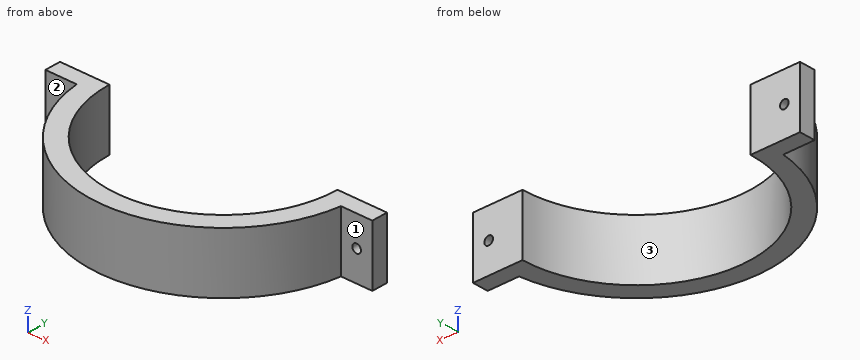
from build123d import *

# Parameters (mm, degrees)
BOSS_EXTRUDE1_DEPTH = 30
SKETCH2_W           = 20
SKETCH2_H           = 8
BOSS_EXTRUDE2_DEPTH = 30
SKETCH3_R           = 2.15265
CUT_EXTRUDE1_DEPTH  = 67.675


with BuildPart() as part:
    # Sketch1 → Boss-Extrude1 (new body)
    with BuildSketch(Plane.XY):
        with BuildLine():
            Line((66.675, 0), (57.15, 0))
            ThreePointArc((57.15, 0), (0, -57.15), (-57.15, 0))
            Line((-57.15, 0), (-66.675, 0))
            ThreePointArc((-66.675, 0), (0, -66.675), (66.675, 0))
        make_face()
    extrude(amount=BOSS_EXTRUDE1_DEPTH)

    # Sketch2 → Boss-Extrude2 (add)
    with BuildSketch(Plane.XY.offset(30)):
        with Locations((71.9125, -4)):
            Rectangle(SKETCH2_W, SKETCH2_H)
        with Locations((-71.9125, -4)):
            Rectangle(SKETCH2_W, SKETCH2_H)
    extrude(amount=-BOSS_EXTRUDE2_DEPTH)

    # Sketch3 → Cut-Extrude1 (cut, through all)
    with BuildSketch(Plane(origin=(0, 0, 0), x_dir=(1, 0, 0), z_dir=(0, 1, 0))):
        with Locations((-74.052910047, -15)):
            Circle(SKETCH3_R)
        with Locations((74.052910047, -15)):
            Circle(SKETCH3_R)
    extrude(amount=-CUT_EXTRUDE1_DEPTH, mode=Mode.SUBTRACT)


solid = part.part
The listing builds one solid part. Answer for the finished solid, in the listing's coordinates (mm). Face numbers are marked on the shaded views. A direction names the side the tool comes from. Round coordinates to 2 decimals unless told otherwise and drop trailing zeros. Write each loop counter-clockwise with the first axis right and the second up, starting at its lowest first coordinate (ties: lowest second). Pieces come first, ordered by that corner, then holes. Notation, with made-up numbers: (-39.5, -24.75) - (-17.5, -24.75) arc R17 cw to (-17.5, -17.75) - close; hole circle Ø4 at (-5, 21). An arc over 180 degrees is marked (long way). Use a Markdown table: item, result. Add a question column.
1. Flat-ended cylindrical pins translate along their axes: P1, Ø10, axis at x = -21.5, z = 25.5, coming from the -Y side; P2, Ø7, axis at x = 74.05, z = 15, coming from the -Y side; P3, Ø1, axis at y = -46.5, z = 21.5, coming from the -X side. Find the tip coordinate at first contact, or state that the pin passes through.
2. The part is cut by section A-A (z = 15). Give the number of separate pieces and of enclosed holes in the cut face, and give its area (3 significant figures).
3. A tool of negligible diameter and unlimited length cuts with its end or side. For the marked faces 1, 2 and 3, from which of +Z, -Z, +X, -X, +Y, -Y can it reach the whole face along a straight path? Write none if from no direction.
4. The part is cut by section B-B (y = -22). Write down the section's boundary in (x, z), and give its area (3 significant figures).
5. Consider line 1 (X direction, y = -2.75, z = 15); line 2 (X direction, y = -3.75, z = 15); line 3 (X direction, y = -29, z = 28.25). Determine where each line is inside the solid, lowest interval first.
6. The part is cut by section D-D (y = -14). Write down the section's boundary in (x, z), and give its area (3 significant figures).
Reported:
| question | item | result |
|---|---|---|
| 1 | P1 | y = -64.6 |
| 1 | P2 | y = -8 |
| 1 | P3 | x = -48.27 |
| 2 | separate pieces | 3 |
| 2 | enclosed holes | 0 |
| 2 | area | 2,030 mm^2 |
| 3 | face 1 | +Z, -Z, +X, -Y |
| 3 | face 2 | +Z, -Z, -X, -Y |
| 3 | face 3 | +Z, -Z, +Y |
| 4 | outline | (-62.94, 0) - (-52.75, 0) - (-52.75, 30) - (-62.94, 30) - close; (52.75, 0) - (62.94, 0) - (62.94, 30) - (52.75, 30) - close |
| 4 | area | 612 mm^2 |
| 5 | line 1 | -81.91 to -76.21, -71.9 to -57.08, 57.08 to 71.9, 76.21 to 81.91 |
| 5 | line 2 | -81.91 to -76.21, -71.9 to -57.03, 57.03 to 71.9, 76.21 to 81.91 |
| 5 | line 3 | -60.04 to -49.25, 49.25 to 60.04 |
| 6 | outline | (-65.19, 0) - (-55.41, 0) - (-55.41, 30) - (-65.19, 30) - close; (55.41, 0) - (65.19, 0) - (65.19, 30) - (55.41, 30) - close |
| 6 | area | 587 mm^2 |
